Here's how the part is built. I have some questions about the finished solid (model axes, mm). Give positions to 0.01 mm unless a question says otherwise; leave off trailing zeros. Order: outer loops, then holes, each group sorted by start corner. A loop starts at its lowest first (then second) coordinate and runs counter-clockwise, first axis right, second up.
from build123d import *

# Parameters (mm, degrees)
BOSS_EXTRUDE1_DEPTH = 0.2794


with BuildPart() as part:
    # Sketch1 → Boss-Extrude1 (new body)
    with BuildSketch(Plane.XY):
        Polygon((-10.9601, 32.766), (-10.9601, 45.466), (10.9601, 45.466), (10.9601, 32.766), (10.9601, -32.766), (-10.9601, -32.766), align=None)
        with BuildLine():
            Line((4.7625, 36.73475), (-4.7625, 36.73475))
            ThreePointArc((-4.7625, 36.73475), (-7.14375, 39.116), (-4.7625, 41.49725))
            Line((-4.7625, 41.49725), (4.7625, 41.49725))
            ThreePointArc((4.7625, 41.49725), (7.14375, 39.116), (4.7625, 36.73475))
        make_face(mode=Mode.SUBTRACT)
    extrude(amount=BOSS_EXTRUDE1_DEPTH)


solid = part.part
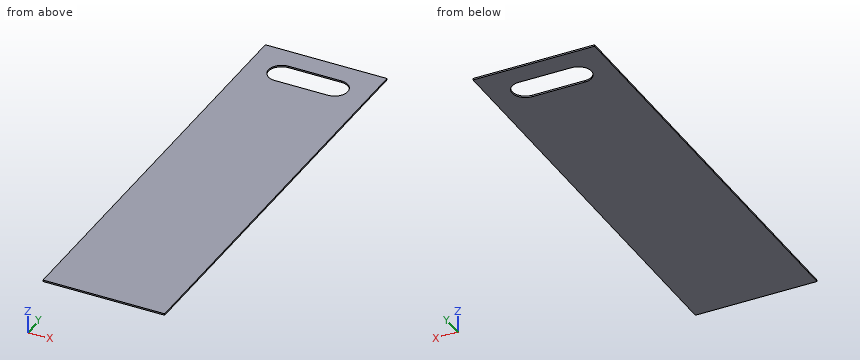
Q1. If we section it at A-A on z = 0.2: List the corners of the cut face in (x, y) for me.
Filled sheet:
outline: (-10.96, -32.77) - (10.96, -32.77) - (10.96, 45.47) - (-10.96, 45.47) - close; hole (-4.76, 36.73) - (4.76, 36.73) arc R2.38 ccw to (4.76, 41.5) - (-4.76, 41.5) arc R2.38 ccw to start
Q2. If we section it at B-B on x = -1.25: List the corners of the cut face in (y, z) for me.
Filled sheet:
outline: (-32.77, 0) - (36.73, 0) - (36.73, 0.28) - (-32.77, 0.28) - close; (41.5, 0) - (45.47, 0) - (45.47, 0.28) - (41.5, 0.28) - close
Q3. If we section it at C-C on x = -5.5: List the corners of the cut face in (y, z) for me.
Filled sheet:
outline: (-32.77, 0) - (36.85, 0) - (36.85, 0.28) - (-32.77, 0.28) - close; (41.38, 0) - (45.47, 0) - (45.47, 0.28) - (41.38, 0.28) - close
Q4. I'm going to push a flat-ended pin straight in: P1, Ø4, axis at x = 0.5, y = 27.5, coming from the -Z side. Where does the tip first touch, or does it pass through?
Filled sheet:
P1: stops at z = 0
Q5. I need wall thicknesses on L1, parallel to Y at x = 1.75, z = 0.1; L2, parallel to Y at x = -6.75, z = 0.1. Which ranges of each line are inside material? Lowest first, please.
Filled sheet:
L1: y = -32.77 to 36.73, 41.5 to 45.47
L2: y = -32.77 to 37.8, 40.43 to 45.47
